```python
from build123d import *

# Parameters (mm, degrees)
F0_W     = 61.5850389004
F0_H     = 58.4090147167
F1_DEPTH = 63.5
F1_TAPER = 6
F2_R     = 8.0775927696
F3_DEPTH = 50.8
F7_D     = 25.4
F7_DEPTH = 50.8
F7_TIP   = 7.6309298617


with BuildPart() as f1:
    # F0 (on Front) → F1 (new body, symmetric)
    with BuildSketch(Plane.XZ):
        with Locations((6.7078769207, 0.9706830606)):
            Rectangle(F0_W, F0_H)
    extrude(amount=F1_DEPTH, both=True, taper=F1_TAPER)

    # F2 (on face) → F3 (join)
    with BuildSketch(Plane(origin=(0, 63.5, 0), x_dir=(-1, 0, 0), z_dir=(0, 1, 0))):
        Circle(F2_R)
    extrude(amount=F3_DEPTH)

    # F4 (on Front) → F5 (revolve)
    with BuildSketch(Plane.XZ):
        Polygon((-52.0598404109, 0), (59.7408004105, 0), (59.7408004105, 23.2562404126), (25.6031993777, 48.4327189624), (-17.0687995851, 48.4327189624), (-52.0598404109, 30.0837587565), align=None)
    revolve(axis=Axis((3.8404799998, 0, 0), (-1, 0, 0)))

    # F7
    with Locations(Plane(origin=(-52.0598404109, 0, 0), x_dir=(0, -1, 0), z_dir=(-1, 0, 0))):
        with Locations((0, 0)):
            Hole(F7_D / 2, depth=F7_DEPTH)
            with Locations((0, 0, -(F7_DEPTH + F7_TIP / 2))):  # 118° drill point
                Cone(0, F7_D / 2, F7_TIP, mode=Mode.SUBTRACT)


solid = f1.part
```
Geometry check sheet. Reference: the model listing, model coordinates, mm. Coordinates: 2 decimals unless noted, no trailing zeros. Loops run counter-clockwise (first coordinate to the right, second up) from the corner with the lowest first, then second, coordinate; pieces in that order, holes last.
Item 1: Sectioned sample at B-B, the plane x = -33.5. Record the boundary of the cut face in (y, z), then the cut area to 3 significant figures.
Item 2: Sectioned sample at A-A, the plane y = 79.5. Record the boundary of the cut face in (x, z), then the cut area to 3 significant figures.
Item 3: Sectioned sample at C-C, the plane x = 36.5. Record the boundary of the cut face in (y, z), then the cut area to 3 significant figures.
Item 4: Go/stop test with flat-tipped pins: pin 1 Ø1 at (y, z) = (20, -37.5) entering from +X; pin 2 Ø6 at (y, z) = (13.5, 31) entering from +X; pin 3 Ø1.5 at (x, z) = (18, 31.5) entering from +Y. Record where each tip stops, or that it passes through.
Item 5: Release check for a two-part mould opening along Z. For faces 1 (the face through (3.968, -0.683, 48.428)), 2 (the face through (-52.06, 0, 13)), 3 (the face through (-26.3, -2.75, -12.4)), 4 (the face through (1.05, 88.54, 8.01)) record: released by +Z, released by -Z, zero draft, split by the parting line, or undercut.
Item 6: Thickness scan on line 1 (Y direction, x = 20.5, z = -20); line 2 (Z direction, x = -38.5, y = 0); line 3 (Y direction, x = -42, z = 0). Record the ranges inside material, lowest first.
Check result:
1. outline: circle Ø79.63 at (0, 0); hole circle Ø25.4 at (0, 0)
1. area: 4,470 mm2
2. outline: circle Ø16.16 at (0, 0)
2. area: 205 mm2
3. outline: circle Ø80.79 at (0, 0)
3. area: 5,130 mm2
4. pin 1: stops at x = 34.33
4. pin 2: stops at x = 49.5
4. pin 3: stops at y = 37.42
5. face 1: released by +Z
5. face 2: zero draft
5. face 3: undercut
5. face 4: split by the parting line
6. line 1: y = -63.5 to 63.5
6. line 2: z = -37.19 to -12.7, 12.7 to 37.19
6. line 3: y = -35.36 to -12.7, 12.7 to 35.36
